The listing builds one solid part. Answer for the finished solid, in the listing's coordinates (mm). A direction names the side the tool comes from. Coordinates: 2 decimals unless noted, no trailing zeros. Order: outer loops, then holes, each group sorted by start corner. A loop starts at its lowest first (then second) coordinate and runs counter-clockwise, first axis right, second up. Notation, with made-up numbers: (24, 76) - (48, 76) arc R26 cw to (48, 110) - close; hole circle Ø4 at (-32, -5.5). An arc over 180 degrees is marked (long way). Use a Markdown table: item, result. Add a question column.
Item 1: The part is cut by section B-B, the plane y = 0. Give the vertices of the cut face in (x, z).
Item 2: Find the intervals of material crossed by line 1 along Y through (x, z) = (-11, 6.25); line 2 along Z through (x, y) = (6, -16.5); line 3 along X through (y, z) = (-12.5, 6), in increasing order.
Item 3: The part is cut by section A-A, the plane x = 0. Give the vertices of the cut face in (y, z).
Item 4: The mould has two halves that part along Y. Classify faces 1 (the flat face through (-11, 10, 2.5)), 2 (the flat face through (19, -13.453, 5)): released by +Y, released by -Y, zero draft, split by the parting line, or undercut.
Item 5: Flat-ended cylindrical pins translate along their axes: P1, Ø1, axis at x = 6, y = -9.5, coming from the -Z side; P2, Ø0.6, axis at x = 19.5, z = 4.5, coming from the +Y side; P3, Ø5, axis at x = -1, z = 7, coming from the -Y side; P4, Ø19, axis at x = -1, y = -7, coming from the +Z side. Find the tip coordinate at first contact, or state that the pin passes through.
Item 6: For faces 3 (the flat face through (19, 11.401, 8)), 4 (the flat face through (-9.721, -12.487, 1.232)), 5 (the flat face through (-11, -12, 9.59)), determine the directions among +Z, -Z, +X, -X, +Y, -Y from which every point of the face is accessible in a straight line to the end or side of a thin tool.
Item 7: The part is cut by section C-C, the plane z = 2. State how many separate pieces and enclosed holes the cut face has, then the cut area to 3 significant figures.
from build123d import *

# Parameters (mm, degrees)
SKETCH2_R                 = 22
BOSS_EXTRUDE1_DEPTH       = 10
SKETCH3_R                 = 21
CUT_EXTRUDE2_DEPTH        = 5.5
SKETCH4_R                 = 1.4
SKETCH4_R_2               = 0.8
BOSS_EXTRUDE2_DEPTH       = 5.09
SKETCH5_R                 = 3
CUT_EXTRUDE3_DEPTH        = 13
BOSS_EXTRUDE3_START       = 5.09
SKETCH6_R                 = 3.5
SKETCH6_R_2               = 3
BOSS_EXTRUDE3_DEPTH       = 5.09
SKETCH18_R                = 0.8
CUT_EXTRUDE7_DEPTH        = 33.557151288
SKETCH20_W                = 10.090622296
SKETCH20_H                = 22.853546686
CUT_EXTRUDE8_DEPTH        = 5
BOSS_EXTRUDE12_DEPTH      = 0.5
BOSS_EXTRUDE12_DEPTH_BACK = 2
FILLET3_R                 = 1.5
CUT_EXTRUDE9_REACH        = 34.68
SKETCH25_W                = 14.266365092
SKETCH25_H                = 28.452518254
BOSS_EXTRUDE14_START      = 5.5
BOSS_EXTRUDE14_DEPTH      = 5.5
BOSS_EXTRUDE15_START      = 5.09
BOSS_EXTRUDE15_DEPTH      = 5.09
SKETCH36_R                = 0.8
CUT_EXTRUDE10_DEPTH       = 2.5


with BuildPart() as part:
    # Sketch2 → Boss-Extrude1 (new body)
    with BuildSketch(Plane.XY):
        Circle(SKETCH2_R)
    extrude(amount=BOSS_EXTRUDE1_DEPTH)

    # Sketch3 → Cut-Extrude2 (cut)
    with BuildSketch(Plane.XY.offset(10)):
        Circle(SKETCH3_R)
    extrude(amount=-CUT_EXTRUDE2_DEPTH, mode=Mode.SUBTRACT)

    # Sketch4 → Boss-Extrude2 (add)
    # profile 1 of 4: a face of its own
    with BuildSketch(Plane.XY.offset(4.5)):
        with Locations((-11, 11)):
            Circle(SKETCH4_R)
        with Locations((-11, 11)):
            Circle(SKETCH4_R_2, mode=Mode.SUBTRACT)
    # profile 2 of 4: a face of its own
    with BuildSketch(Plane.XY.offset(4.5)):
        with Locations((10, 11)):
            Circle(SKETCH4_R)
        with Locations((10, 11)):
            Circle(SKETCH4_R_2, mode=Mode.SUBTRACT)
    # profile 3 of 4: a face of its own
    with BuildSketch(Plane.XY.offset(4.5)):
        with Locations((10, -11.015029648)):
            Circle(SKETCH4_R)
        with Locations((10, -11.015029648)):
            Circle(SKETCH4_R_2, mode=Mode.SUBTRACT)
    # profile 4 of 4: a face of its own
    with BuildSketch(Plane.XY.offset(4.5)):
        with Locations((-11, -11.015029648)):
            Circle(SKETCH4_R)
        with Locations((-11, -11.015029648)):
            Circle(SKETCH4_R_2, mode=Mode.SUBTRACT)
    extrude(amount=BOSS_EXTRUDE2_DEPTH)

    # Sketch5 → Cut-Extrude3 (cut)
    with BuildSketch(Plane.XY.offset(4.5)):
        Circle(SKETCH5_R)
    extrude(amount=-CUT_EXTRUDE3_DEPTH, mode=Mode.SUBTRACT)

    # Sketch6 → Boss-Extrude3 (add)
    with BuildSketch(Plane.XY.offset(4.5).offset(BOSS_EXTRUDE3_START)):
        Circle(SKETCH6_R)
        Circle(SKETCH6_R_2, mode=Mode.SUBTRACT)
    extrude(amount=-BOSS_EXTRUDE3_DEPTH)

    # Sketch18 → Cut-Extrude7 (cut, through all)
    with BuildSketch(Plane.XY.offset(9.59)):
        with Locations((-11, 11)):
            Circle(SKETCH18_R)
        with Locations((10, 11)):
            Circle(SKETCH18_R)
        with Locations((10, -11.015029648)):
            Circle(SKETCH18_R)
        with Locations((-11, -11.015029648)):
            Circle(SKETCH18_R)
    extrude(amount=-CUT_EXTRUDE7_DEPTH, mode=Mode.SUBTRACT)

    # Sketch20 → Cut-Extrude8 (cut)
    with BuildSketch(Plane.XY.offset(10)):
        with Locations((22.416150926, -0.026114621)):
            Rectangle(SKETCH20_W, SKETCH20_H)
    extrude(amount=-CUT_EXTRUDE8_DEPTH, mode=Mode.SUBTRACT)

    # Sketch24 → Boss-Extrude12 (add, two sides: drawn at the far end of the back side and taken through both)
    with BuildSketch(Plane(origin=(20.459151462, 0, 0), x_dir=(0, 0, -1), z_dir=(1, 0, 0)).offset(-BOSS_EXTRUDE12_DEPTH_BACK)):
        Polygon((-10, 11.400658722), (-5, 11.400658722), (-5, -11.452887964), (-10, -11.452887964), (-10, -13.452887964), (0, -13.452887964), (0, 13.400658722), (-10, 13.400658722), align=None)
    extrude(amount=BOSS_EXTRUDE12_DEPTH + BOSS_EXTRUDE12_DEPTH_BACK)

    # Fillet3
    # the kernel refuses this fillet: 1.5 mm, written as the material it adds along each edge
    with BuildSketch(Plane(origin=(18.459151462, -11.96911556, 10), x_dir=(-0.5904449589770525, -0.8070779085184941, 0), z_dir=(0, 0, -1))) as fillet3_piece_1:
        with BuildLine():
            CenterArc((2.562692726, -1.497618907), FILLET3_R, 93.228774065, 62.292501853)
            Line((1.197519929, -0.876085936), (1.170216473, -0.863655277))
            ThreePointArc((1.170216473, -0.863655277), (0.581046616, -0.462255305), (-0.017713349, -0.024212337))
            Line((-0.017713349, -0.024212337), (0.001689688, 0.029952378))
            ThreePointArc((0.001689688, 0.029952378), (1.239104175, -0.004922699), (2.476518663, 0.029952378))
            Line((2.476518663, 0.029952378), (2.47820835, 0))
        make_face()
    extrude(amount=10)
    with BuildSketch(Plane(origin=(18.459151462, 11.96911556, 10), x_dir=(0, 1, 0), z_dir=(0, 0, -1))) as fillet3_piece_2:
        with BuildLine():
            CenterArc((2.907499122, -0.267495804), FILLET3_R, 169.727466674, 60.997217104)
            Line((1.957927972, -1.428665314), (1.938936549, -1.451888704))
            ThreePointArc((1.938936549, -1.451888704), (0.980970205, -0.711583215), (-0.016321521, -0.02517157))
            Line((-0.016321521, -0.02517157), (0, 0.03))
            ThreePointArc((0, 0.03), (0.715771581, 0.03), (1.402024043, 0.005349916))
            Line((1.402024043, 0.005349916), (1.431543163, 0))
        make_face()
    extrude(amount=10)

    # Sketch25 → Cut-Extrude9 (cut, up to next)
    with BuildSketch(Plane.XY.offset(10), mode=Mode.PRIVATE) as cut_extrude9_sk1:
        with Locations((27.566848105, 0.101683084)):
            Rectangle(SKETCH25_W, SKETCH25_H)
    cut_extrude9_tool1 = extrude(cut_extrude9_sk1.sketch, amount=-CUT_EXTRUDE9_REACH, mode=Mode.PRIVATE) & part.part
    add(cut_extrude9_tool1.solids().sort_by_distance((27.566848, 0.101683, 10))[0], mode=Mode.SUBTRACT)

    # Sketch30 → Boss-Extrude14 (add)
    with BuildSketch(Plane.XY.offset(4.5).offset(BOSS_EXTRUDE14_START)):
        with BuildLine():
            ThreePointArc((2.255465854, -20.878526619), (-0.002066694, -17.580176404), (-2.260374676, -20.877995745))
            ThreePointArc((-2.260374676, -20.877995745), (-0.002468723, -20.999999855), (2.255465854, -20.878526619))
        make_face()
        with BuildLine():
            ThreePointArc((-2.203022296, 20.884125377), (-0.002233305, 17.624620846), (2.197729558, 20.884683019))
            ThreePointArc((2.197729558, 20.884683019), (-0.002661017, 20.999999831), (-2.203022296, 20.884125377))
        make_face()
        with BuildLine():
            ThreePointArc((-20.883881485, -2.205333104), (-17.630224728, -0.00211959), (-20.884411153, 2.200311519))
            ThreePointArc((-20.884411153, 2.200311519), (-20.999999848, -0.002524721), (-20.883881485, -2.205333104))
        make_face()
    extrude(amount=-BOSS_EXTRUDE14_DEPTH)

    # Sketch33 → Boss-Extrude15 (add)
    with BuildSketch(Plane.XY.offset(4.5).offset(BOSS_EXTRUDE15_START)):
        with BuildLine():
            Line((16.263091014, 11.640956604), (17.076245565, 12.223004435))
            ThreePointArc((17.076245565, 12.223004435), (10.565400997, 18.148617076), (2.197729558, 20.884683019))
            ThreePointArc((2.197729558, 20.884683019), (2.280216576, 20.643620919), (2.336378022, 20.395103458))
            ThreePointArc((2.336378022, 20.395103458), (-0.256894976, 17.638295394), (-2.203022296, 20.884125377))
            ThreePointArc((-2.203022296, 20.884125377), (-14.850206089, 14.848278658), (-20.884411153, 2.200311519))
            ThreePointArc((-20.884411153, 2.200311519), (-17.630224728, -0.00211959), (-20.883881485, -2.205333104))
            ThreePointArc((-20.883881485, -2.205333104), (-14.868800585, -14.82965843), (-2.260374676, -20.877995745))
            ThreePointArc((-2.260374676, -20.877995745), (-0.002066694, -17.580176404), (2.255465854, -20.878526619))
            ThreePointArc((2.255465854, -20.878526619), (10.376578748, -18.257234552), (16.784176211, -12.621070831))
            Line((16.784176211, -12.621070831), (15.984929724, -12.020067458))
            ThreePointArc((15.984929724, -12.020067458), (10.430037734, -17.065002575), (3.406904238, -19.707688944))
            ThreePointArc((3.406904238, -19.707688944), (-0.001949136, -16.580176411), (-3.411537746, -19.70688738))
            ThreePointArc((-3.411537746, -19.70688738), (-14.159639755, -14.1246098), (-19.715277269, -3.362713518))
            ThreePointArc((-19.715277269, -3.362713518), (-16.630224735, -0.001999366), (-19.716085262, 3.35797289))
            ThreePointArc((-19.716085262, 3.35797289), (-14.144029066, 14.140241928), (-3.36325256, 19.71518532))
            ThreePointArc((-3.36325256, 19.71518532), (-0.00210659, 16.624620854), (3.358256029, 19.716037037))
            ThreePointArc((3.358256029, 19.716037037), (10.609007774, 16.954319628), (16.263091014, 11.640956604))
        make_face()
    extrude(amount=-BOSS_EXTRUDE15_DEPTH)

    # Sketch36 → Cut-Extrude10 (cut)
    # profile 1 of 4: a face of its own
    with BuildSketch(Plane(origin=(0, 0, 0), x_dir=(-1, 0, 0), z_dir=(0, 0, -1))):
        Polygon((-7.74833395, 11), (-8.874166975, 12.95), (-11.125833025, 12.95), (-12.25166605, 11), (-11.125833025, 9.05), (-8.874166975, 9.05), align=None)
        with Locations((-10, 11)):
            Circle(SKETCH36_R, mode=Mode.SUBTRACT)
    # profile 2 of 4: a face of its own
    with BuildSketch(Plane(origin=(0, 0, 0), x_dir=(-1, 0, 0), z_dir=(0, 0, -1))):
        Polygon((12.514649012, 12.666084743), (10.314452793, 13.144766893), (8.799803782, 11.47868215), (9.485350988, 9.333915257), (11.685547207, 8.855233107), (13.200196218, 10.52131785), align=None)
        with Locations((11, 11)):
            Circle(SKETCH36_R, mode=Mode.SUBTRACT)
    # profile 3 of 4: a face of its own
    with BuildSketch(Plane(origin=(0, 0, 0), x_dir=(-1, 0, 0), z_dir=(0, 0, -1))):
        Polygon((13.122597825, -10.263645278), (11.41058096, -8.801113824), (9.287983135, -9.552498195), (8.877402175, -11.766414018), (10.58941904, -13.228945472), (12.712016865, -12.477561101), align=None)
        with Locations((11, -11.015029648)):
            Circle(SKETCH36_R, mode=Mode.SUBTRACT)
    # profile 4 of 4: a face of its own
    with BuildSketch(Plane(origin=(0, 0, 0), x_dir=(-1, 0, 0), z_dir=(0, 0, -1))):
        Polygon((-8.492299155, -9.342654641), (-10.694468818, -8.873134912), (-12.202169663, -10.545509919), (-11.507700845, -12.687404655), (-9.305531182, -13.156924384), (-7.797830337, -11.484549377), align=None)
        with Locations((-10, -11.015029648)):
            Circle(SKETCH36_R, mode=Mode.SUBTRACT)
    extrude(amount=-CUT_EXTRUDE10_DEPTH, mode=Mode.SUBTRACT)


solid = part.part
Solution:
| question | item | result |
|---|---|---|
| 1 | outline | (-22, 0) - (-3, 0) - (-3, 9.59) - (-3.5, 9.59) - (-3.5, 4.5) - (-16.63, 4.5) - (-16.63, 9.59) - (-17.63, 9.59) - (-17.63, 10) - (-22, 10) - close; (3, 0) - (20.43, 0) - (20.43, 5) - (18.46, 5) - (18.46, 4.5) - (3.5, 4.5) - (3.5, 9.59) - (3, 9.59) - close |
| 2 | line 1 | y = -19.05 to -16.7, -12.42 to -11.82, -10.22 to -9.62, 9.6 to 10.2, 11.8 to 12.4, 16.7 to 19.05 |
| 2 | line 2 | z = 0 to 4.5 |
| 2 | line 3 | x = -18.1 to -15.61, 15.61 to 16.62, 16.87 to 20.43 |
| 3 | outline | (-22, 0) - (-3, 0) - (-3, 9.59) - (-3.5, 9.59) - (-3.5, 4.5) - (-16.58, 4.5) - (-16.58, 9.59) - (-17.58, 9.59) - (-17.58, 10) - (-22, 10) - close; (3, 0) - (22, 0) - (22, 10) - (17.62, 10) - (17.62, 9.59) - (16.62, 9.59) - (16.62, 4.5) - (3.5, 4.5) - (3.5, 9.59) - (3, 9.59) - close |
| 4 | face 1 | undercut |
| 4 | face 2 | released by -Y |
| 5 | P1 | stops at z = 0 |
| 5 | P2 | stops at y = 13.4 |
| 5 | P3 | stops at y = -22 |
| 5 | P4 | stops at z = 9.59 |
| 6 | face 3 | +Z, +X |
| 6 | face 4 | -Z |
| 6 | face 5 | +Z |
| 7 | separate pieces | 1 |
| 7 | enclosed holes | 5 |
| 7 | area | 1,440 mm2 |
